Geometry check sheet. Reference: the model listing, model coordinates, mm. A direction names the side the tool comes from. Round coordinates to 2 decimals unless told otherwise and drop trailing zeros. Loops run counter-clockwise (first coordinate to the right, second up) from the corner with the lowest first, then second, coordinate; pieces in that order, holes last. Notation, with made-up numbers: (-11, 48.25) -> (19, 48.25) arc R34 ccw to (19, 83.25) -> close; hole circle Ø11 at (-12, 60). An arc over 180 degrees is marked (long way). Use one line per item in the form item = value.
from build123d import *
from build123d.topology import SkipClean

# Parameters (mm, degrees)
BOSS_EXTRUDE1_DEPTH = 4
BOSS_EXTRUDE2_DEPTH = 2.5
SKETCH3_R           = 7.95
CUT_EXTRUDE1_DEPTH  = 9.25
SKETCH4_R           = 1.65
CUT_EXTRUDE2_DEPTH  = 9.25
CUT_EXTRUDE3_DEPTH  = 3.25
FILLET1_R           = 2.38125
CHAMFER1_SIZE       = 3.5
CHAMFER1_SIZE2      = 2.020725942
BOSS_EXTRUDE4_DEPTH = 4
BOSS_EXTRUDE5_START = 2.25
SKETCH11_R          = 11.95
BOSS_EXTRUDE5_DEPTH = 2.25
CUT_EXTRUDE4_START  = -2.25
SKETCH12_R          = 7.95
CUT_EXTRUDE4_DEPTH  = 2.25
FILLET5_R           = 2.38


with BuildPart() as part:
    # Sketch1 → Boss-Extrude1 (new body)
    with BuildSketch(Plane(origin=(0, 0, 0), x_dir=(1, 0, 0), z_dir=(0, 1, 0))):
        with BuildLine():
            Line((-13.29118379, 20.889836125), (-0.68999579, 20.889836125))
            Line((-0.68999579, 20.889836125), (-0.68999579, 26.09210312))
            Line((-0.68999579, 26.09210312), (12.01000421, 26.09210312))
            Line((12.01000421, 26.09210312), (12.01000421, -28.90789688))
            Line((12.01000421, -28.90789688), (-0.68999579, -28.90789688))
            Line((-0.68999579, -28.90789688), (-0.68999579, -23.705629885))
            Line((-0.68999579, -23.705629885), (-13.29118379, -23.705629885))
            ThreePointArc((-13.29118379, -23.705629885), (-35.588916795, -1.40789688), (-13.29118379, 20.889836125))
        make_face()
    extrude(amount=BOSS_EXTRUDE1_DEPTH)

    # Sketch2 → Boss-Extrude2 (add)
    with BuildSketch(Plane(origin=(0, 4, 0), x_dir=(1, 0, 0), z_dir=(0, 1, 0))):
        with BuildLine():
            Line((-13.29118379, 20.889836125), (-0.68999579, 20.889836125))
            Line((-0.68999579, 20.889836125), (-0.68999579, 16.987726462))
            ThreePointArc((-0.68999579, 16.987726462), (9.006549215, -1.40789688), (-0.68999579, -19.803520222))
            Line((-0.68999579, -19.803520222), (-0.68999579, -23.705629885))
            Line((-0.68999579, -23.705629885), (-13.29118379, -23.705629885))
            ThreePointArc((-13.29118379, -23.705629885), (-35.588916795, -1.40789688), (-13.29118379, 20.889836125))
        make_face()
    extrude(amount=BOSS_EXTRUDE2_DEPTH)

    # Sketch3 → Cut-Extrude1 (cut)
    with BuildSketch(Plane.XZ):
        with Locations(Location((-13.29118379, 1.40789688, 0), (0, 0, 270))):
            Circle(SKETCH3_R)
    extrude(amount=-CUT_EXTRUDE1_DEPTH, mode=Mode.SUBTRACT)

    # Sketch4 → Cut-Extrude2 (cut)
    with BuildSketch(Plane.XZ):
        with Locations(Location((3.31000421, 24.40789688, 0), (0, 0, 270))):
            Circle(SKETCH4_R)
        with Locations(Location((3.310004206, -21.59210312, 0), (0, 0, 270))):
            Circle(SKETCH4_R)
    extrude(amount=-CUT_EXTRUDE2_DEPTH, mode=Mode.SUBTRACT)

    # Sketch5 → Cut-Extrude3 (cut)
    with BuildSketch(Plane.XZ):
        with BuildLine():
            ThreePointArc((-20.917233099, -7.792422241), (-25.24118379, 1.40789688), (-20.917233099, 10.608216001))
            Line((-20.917233099, 10.608216001), (-24.193916765, 16.291878661))
            ThreePointArc((-24.193916765, 16.291878661), (-31.74118379, 1.40789688), (-24.193916765, -13.476084902))
            Line((-24.193916765, -13.476084902), (-20.917233099, -7.792422241))
        make_face()
        with BuildLine():
            Line((-20.729723635, 18.291931497), (-17.445869217, 12.612408873))
            ThreePointArc((-17.445869217, 12.612408873), (-7.31618379, 11.756900455), (-1.510449053, 3.412089752))
            Line((-1.510449053, 3.412089752), (5.05008903, 3.407949716))
            ThreePointArc((5.05008903, 3.407949716), (-4.06618379, 17.38606558), (-20.729723635, 18.291931497))
        make_face()
        with BuildLine():
            ThreePointArc((-1.510449053, -0.596295992), (-7.31618379, -8.941106696), (-17.445869217, -9.796615113))
            Line((-17.445869217, -9.796615113), (-20.729723635, -15.476137738))
            ThreePointArc((-20.729723635, -15.476137738), (-4.06618379, -14.57027182), (5.05008903, -0.592155956))
            Line((5.05008903, -0.592155956), (-1.510449053, -0.596295992))
        make_face()
    extrude(amount=-CUT_EXTRUDE3_DEPTH, mode=Mode.SUBTRACT)

    # Fillet1
    fillet1_edges = [part.edges().sort_by_distance(p)[0] for p in [
        (-20.917233099, 1.625, 10.608216001),
        (-20.917233099, 1.625, -7.792422241),
        (-24.193916765, 1.625, -13.476084902),
        (-24.193916765, 1.625, 16.291878661),
        (5.05008903, 1.625, 3.407949716),
        (-1.510449053, 1.625, 3.412089752),
        (-17.445869217, 1.625, 12.612408873),
        (-20.729723635, 1.625, 18.291931497),
        (-17.445869217, 1.625, -9.796615113),
        (-1.510449053, 1.625, -0.596295992),
        (5.05008903, 1.625, -0.592155956),
        (-20.729723635, 1.625, -15.476137738),
    ]]
    fillet(fillet1_edges, radius=FILLET1_R)

    # Chamfer1
    chamfer1_edges = [part.edges().sort_by_distance(p)[0] for p in [
        (12.01000421, 0, 1.40789688),
    ]]
    chamfer1_side = [part.faces().sort_by_distance(p)[0] for p in [
        (-3.702499267, 0, 18.015985651),
    ]]
    chamfer(chamfer1_edges, length=CHAMFER1_SIZE, length2=CHAMFER1_SIZE2, reference=chamfer1_side[0])

    # Sketch10 → Boss-Extrude4 (add)
    with BuildSketch(Plane.XZ):
        with BuildLine():
            Line((-0.68999579, -22.889836125), (-13.29118379, -22.889836125))
            ThreePointArc((-13.29118379, -22.889836125), (-37.588916795, 1.40789688), (-13.29118379, 25.705629885))
            Line((-13.29118379, 25.705629885), (-0.68999579, 25.705629885))
            Line((-0.68999579, 25.705629885), (-0.68999579, 23.705629885))
            Line((-0.68999579, 23.705629885), (-13.29118379, 23.705629885))
            ThreePointArc((-13.29118379, 23.705629885), (-35.588916795, 1.40789688), (-13.29118379, -20.889836125))
            Line((-13.29118379, -20.889836125), (-0.68999579, -20.889836125))
            Line((-0.68999579, -20.889836125), (-0.68999579, -22.889836125))
        make_face()
    extrude(amount=-BOSS_EXTRUDE4_DEPTH)

    # Sketch11 → Boss-Extrude5 (add)
    with SkipClean():  # the faces are left unmerged after this step: merging them gives an invalid solid
        with BuildSketch(Plane.XZ.offset(BOSS_EXTRUDE5_START)):
            with Locations(Location((-13.29118379, 1.40789688, 0), (0, 0, 270))):
                Circle(SKETCH11_R)
        extrude(amount=-BOSS_EXTRUDE5_DEPTH)

    # Sketch12 → Cut-Extrude4 (cut)
    with SkipClean():  # the faces are left unmerged after this step: merging them gives an invalid solid
        with BuildSketch(Plane(origin=(0, 0, 0), x_dir=(1, 0, 0), z_dir=(0, 1, 0)).offset(CUT_EXTRUDE4_START)):
            with Locations(Location((-13.29118379, -1.40789688, 0), (0, 0, 270))):
                Circle(SKETCH12_R)
        extrude(amount=CUT_EXTRUDE4_DEPTH, mode=Mode.SUBTRACT)

    # Fillet5
    fillet5_edges = [part.edges().sort_by_distance(p)[0] for p in [
        (-0.68999579, 5.25, 19.803520222),
        (-0.68999579, 5.25, -16.987726462),
    ]]
    fillet(fillet5_edges, radius=FILLET5_R)


solid = part.part
1. Section check A-A (y = 5). Record the boundary of the cut face in (x, z).
Return value:
outline = (-13.29, -20.89) -> (-0.69, -20.89) -> (-0.69, -18.2) arc R2.38 cw to (0.25, -16.31) arc R22.3 ccw to (0.25, 19.13) arc R2.38 cw to (-0.69, 21.02) -> (-0.69, 23.71) -> (-13.29, 23.71) arc R22.3 ccw to start; hole circle Ø15.9 at (-13.29, 1.41)
2. Material ranges on line 1 along Z through (x, y) = (-13, 0.5); line 2 along X through (y, z) = (2, -4.5); line 3 along Z through (x, y) = (-18.5, 3), recorded low to high.
Return value:
line_1 = -22.89 to -17.04, -10.54 to -6.54, 9.35 to 13.35, 19.86 to 25.71
line_2 = -36.86 to -30.77, -23.68 to -18.61, -7.97 to -2.9, 4.19 to 11.97
line_3 = -22.32 to -16.18, -11.62 to -4.6, 7.41 to 14.44, 19 to 25.14
3. Mould release check, pull along Z, two halves, no side actions. Record for faces 1 (the flat face through (-0.69, 2, 27)), 2 (the flat face through (6, 2, -26.092)), 3 (the cylindrical face through (3.383, 1.972, -19.944)), 4 (the flat face through (6, 2, 28.908)): released by +Z, released by -Z, zero draft, split by the parting line, or undercut.
Return value:
face_1 = zero draft
face_2 = released by -Z
face_3 = undercut
face_4 = released by +Z
4. Section check C-C (z = -15). Record the boundary of the cut face in (x, y), then the cut area to 3 significant figures.
Return value:
outline = (-31.21, 0) -> (-19.46, 0) -> (-19.46, 3.25) -> (-4.85, 3.25) -> (-4.85, 0) -> (8.51, 0) -> (12.01, 2.02) -> (12.01, 4) -> (1.81, 4) -> (1.81, 6.5) -> (-28.39, 6.5) -> (-28.39, 4) -> (-31.21, 4) -> close
area = 197 mm2
5. Gauge pin test, flat ends, axial feed: pin 1 (0.8 mm diameter, centred on y = 5, z = -20, fed in from +X); pin 2 (3 mm diameter, centred on x = -4.5, y = 5, fed in from -Z); pin 3 (5.5 mm diameter, centred on x = 3.31, z = 24.41, fed in from +Y). Record the tip position at first contact, or that the pin passes through.
Return value:
pin_1 = -0.69
pin_2 = -22.89
pin_3 = 4
6. Section check D-D (x = -32.5). Record the boundary of the cut face in (y, z), then the cut area to 3 significant figures.
Return value:
outline = (0, -13.47) -> (4, -13.47) -> (4, -9.92) -> (6.5, -9.92) -> (6.5, 12.73) -> (4, 12.73) -> (4, 16.29) -> (0, 16.29) -> close
area = 176 mm2
7. Section check B-B (z = 2). Record the boundary of the cut face in (x, y).
Return value:
outline = (-37.58, 0) -> (-31.73, 0) -> (-31.73, 3.25) -> (-25.23, 3.25) -> (-25.23, -2.25) -> (-21.22, -2.25) -> (-21.22, 6.5) -> (-35.58, 6.5) -> (-35.58, 4) -> (-37.58, 4) -> close; (-5.36, -2.25) -> (-1.36, -2.25) -> (-1.36, 0) -> (8.51, 0) -> (12.01, 2.02) -> (12.01, 4) -> (9, 4) -> (9, 6.5) -> (-5.36, 6.5) -> close
8. Tool access check on faces 5 (the cylindrical face through (-37.583, 1.972, 0.874)), 6 (the flat face through (-27, 3.25, 2)), 7 (the cylindrical face through (-0.437, 5.268, 19.949)), 8 (the flat face through (-7, 5, 23.706)). Record the directions out of +Z, -Z, +X, -X, +Y, -Y that give a thin tool (end or side, any length) a straight path to the whole face; none if there is none.
Return value:
face_5 = -X, +Y, -Y
face_6 = -Y
face_7 = +Z, +X, +Y
face_8 = +Z, +X, -X, +Y
